Geometry: final body of the model. Coordinates: model frame, mm. Face numbers are marked on the shaded views. A direction names the side the tool comes from. Round coordinates to 2 decimals unless told otherwise and drop trailing zeros. Write each loop counter-clockwise with the first axis right and the second up, starting at its lowest first coordinate (ties: lowest second). Pieces come first, ordered by that corner, then holes. Notation, with made-up numbers: M -23,-3.75 L -5,-3.75 A24 ccw -5,31.25 Z; hole C -37,36 d5. An arc over 180 degrees is marked long. Use one line per item in the form item = value. Start each with the question number.
Item 1: Section query B-B (z = -105). Return loops of the section in (x, y).
Item 2: Pull-direction query (Z, two-part tool) for the marked faces 3, 4, 5 and 6; classes: pulls with the +Z half, pulls with the -Z half, needs draft (parallel to the pull), parting line crosses it, or undercut.
Item 3: Section query C-C (x = -43). Return loops of the section in (y, z), and give its area (3 significant figures).
Item 4: Pin query (flat end, axial travel): pin 1 Ø13.5 at (x, y) = (45, 0) entering from -Z. Return the tip coordinate at first contact, or that it passes through.
Item 5: Ray query, probe 1 along Z at (x, y) = (54.5, -0.75); probe 2 along Y at (x, z) = (-45, -16.25); probe 3 along Z at (x, y) = (19.5, 13.75). Return the intervals inside material, ascending.
Item 6: Section query A-A (x = 34). Return loops of the section in (y, z), and give its area (3 significant figures).
Item 7: Reachability of the marked faces 1 and 2 from +Z, -Z, +X, -X, +Y, -Y: full face, straight path, thin tool, end or side. Return the list, or none.
Item 8: Section query D-D (y = 0). State how many separate pieces and enclosed holes the cut face has, and give its area (3 significant figures).
from build123d import *

# Parameters (mm, degrees)
BOSS_EXTRUDE1_DEPTH      = 15
BOSS_EXTRUDE1_DEPTH_BACK = 15
SKETCH2_R                = 4.25
CUT_EXTRUDE1_DEPTH       = 120
SKETCH3_R                = 7.5
CUT_EXTRUDE2_DEPTH       = 142
FILLET1_R                = 3


with BuildPart() as part:
    # Sketch1 → Boss-Extrude1 (new, two sides: drawn at the far end of the back side and taken through both)
    with BuildSketch(Plane(origin=(0, 0, 0), x_dir=(1, 0, 0), z_dir=(0, 1, 0)).offset(-BOSS_EXTRUDE1_DEPTH_BACK)):
        with BuildLine():
            Line((-75, 0), (75, 0))
            ThreePointArc((75, 0), (96.213203436, 8.786796564), (105, 30))
            Line((105, 30), (105, 125))
            ThreePointArc((105, 125), (96.213203436, 146.213203436), (75, 155))
            Line((75, 155), (-75, 155))
            ThreePointArc((-75, 155), (-96.213203436, 146.213203436), (-105, 125))
            Line((-105, 125), (-105, 30))
            ThreePointArc((-105, 30), (-96.213203436, 8.786796564), (-75, 0))
        make_face()
        with BuildLine():
            Line((-75, 140), (75, 140))
            ThreePointArc((75, 140), (85.606601718, 135.606601718), (90, 125))
            Line((90, 125), (90, 35))
            ThreePointArc((90, 35), (85.606601718, 24.393398282), (75, 20))
            Line((75, 20), (-75, 20))
            ThreePointArc((-75, 20), (-85.606601718, 24.393398282), (-90, 35))
            Line((-90, 35), (-90, 125))
            ThreePointArc((-90, 125), (-85.606601718, 135.606601718), (-75, 140))
        make_face(mode=Mode.SUBTRACT)
    extrude(amount=BOSS_EXTRUDE1_DEPTH + BOSS_EXTRUDE1_DEPTH_BACK)

    # Sketch2 → Cut-Extrude1 (cut)
    with BuildSketch(Plane.XY):
        with Locations((45, 0)):
            Circle(SKETCH2_R)
        with Locations((-45, 0)):
            Circle(SKETCH2_R)
    extrude(amount=-CUT_EXTRUDE1_DEPTH, mode=Mode.SUBTRACT)

    # Sketch3 → Cut-Extrude2 (cut)
    with BuildSketch(Plane(origin=(0, 0, -155), x_dir=(-1, 0, 0), z_dir=(0, 0, -1))):
        with Locations((45, 0)):
            Circle(SKETCH3_R)
        with Locations((-45, 0)):
            Circle(SKETCH3_R)
    extrude(amount=-CUT_EXTRUDE2_DEPTH, mode=Mode.SUBTRACT)

    # Fillet1
    fillet1_edges = [part.edges().sort_by_distance(p)[0] for p in [
        (-96.213203436, -15, -146.213203436),
        (-105, -15, -77.5),
        (-96.213203436, -15, -8.786796564),
        (0, -15, 0),
        (-85.606601718, -15, -135.606601718),
        (0, -15, -140),
        (85.606601718, -15, -135.606601718),
        (90, -15, -80),
        (96.213203436, -15, -8.786796564),
        (85.606601718, -15, -24.393398282),
        (0, -15, -20),
        (-85.606601718, -15, -24.393398282),
        (-90, -15, -80),
        (105, -15, -77.5),
        (96.213203436, 15, -146.213203436),
        (0, 15, -155),
        (-96.213203436, 15, -146.213203436),
        (-105, 15, -77.5),
        (-96.213203436, 15, -8.786796564),
        (0, 15, 0),
        (96.213203436, 15, -8.786796564),
        (105, 15, -77.5),
        (96.213203436, -15, -146.213203436),
        (-85.606601718, 15, -135.606601718),
        (-90, 15, -80),
        (-85.606601718, 15, -24.393398282),
        (0, 15, -20),
        (85.606601718, 15, -24.393398282),
        (90, 15, -80),
        (85.606601718, 15, -135.606601718),
        (0, 15, -140),
        (0, -15, -155),
    ]]
    fillet(fillet1_edges, radius=FILLET1_R)


solid = part.part
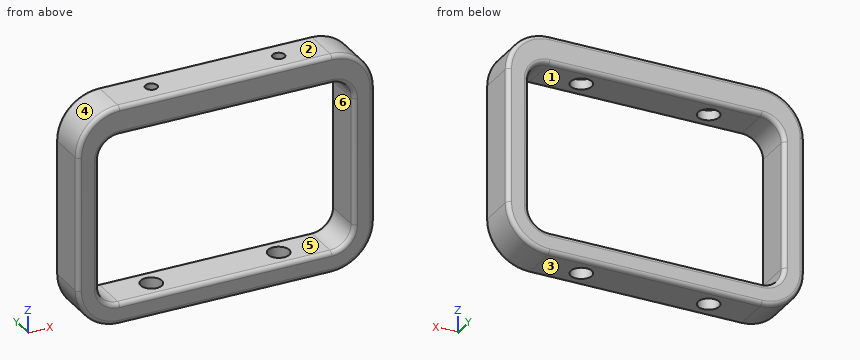
Working result:
q1.outline = M -105,-12 A3 ccw -102,-15 L -93,-15 A3 ccw -90,-12 L -90,12 A3 ccw -93,15 L -102,15 A3 ccw -105,12 Z; M 90,-12 A3 ccw 93,-15 L 102,-15 A3 ccw 105,-12 L 105,12 A3 ccw 102,15 L 93,15 A3 ccw 90,12 Z
q2.face_3 = pulls with the -Z half
q2.face_4 = pulls with the +Z half
q2.face_5 = undercut
q2.face_6 = undercut
q3.outline = M -15,-152 A3 ccw -12,-155 L -7.23,-155 L -7.23,-140 L -12,-140 A3 ccw -15,-143 Z; M -15,-17 A3 ccw -12,-20 L -7.23,-20 L -7.23,-13 L -3.75,-13 L -3.75,0 L -12,0 A3 ccw -15,-3 Z; M 3.75,-13 L 7.23,-13 L 7.23,-20 L 12,-20 A3 ccw 15,-17 L 15,-3 A3 ccw 12,0 L 3.75,0 Z; M 7.23,-155 L 12,-155 A3 ccw 15,-152 L 15,-143 A3 ccw 12,-140 L 7.23,-140 Z
q3.area = 619 mm²
q4.pin_1 = -13
q5.probe_1 = -155 to -140, -20 to 0
q5.probe_2 = -15 to -7.5, 7.5 to 15
q5.probe_3 = -154.44 to -140.56, -19.44 to -0.56
q6.outline = M -15,-152 A3 ccw -12,-155 L 12,-155 A3 ccw 15,-152 L 15,-143 A3 ccw 12,-140 L -12,-140 A3 ccw -15,-143 Z; M -15,-17 A3 ccw -12,-20 L 12,-20 A3 ccw 15,-17 L 15,-3 A3 ccw 12,0 L -12,0 A3 ccw -15,-3 Z
q6.area = 1,030 mm²
q7.face_1 = +Y, -Y
q7.face_2 = +Z, +X, -X, +Y, -Y
q8.separate_pieces = 4
q8.enclosed_holes = 0
q8.area = 9,490 mm²
